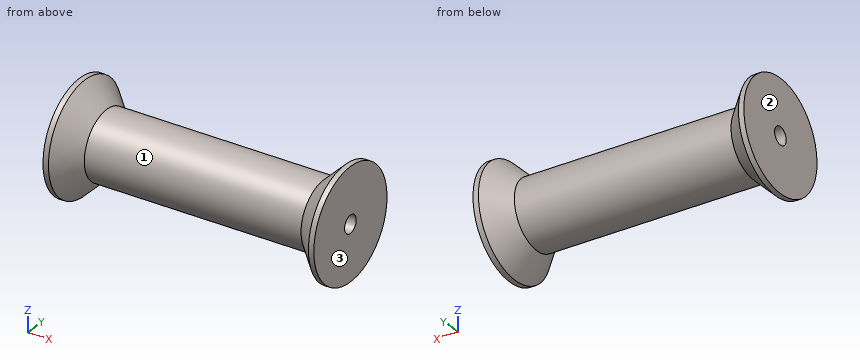
```python
from build123d import *


with BuildPart() as part:
    # Sketch1 → Revolve1 (revolve)
    with BuildSketch(Plane.XY, mode=Mode.PRIVATE) as revolve1_sk:
        with BuildLine():
            Line((0, 3.25), (10, 3.25))
            ThreePointArc((10, 3.25), (20.351145141, 7.537584704), (31.459292144, 9))
            Line((31.459292144, 9), (68.540707856, 9))
            ThreePointArc((68.540707856, 9), (79.648854859, 7.537584704), (90, 3.25))
            Line((90, 3.25), (100, 3.25))
            Line((100, 3.25), (100, 20.5))
            Line((100, 20.5), (98, 20.5))
            Line((98, 20.5), (90, 12.5))
            Line((90, 12.5), (10, 12.5))
            Line((10, 12.5), (2, 20.5))
            Line((2, 20.5), (0, 20.5))
            Line((0, 20.5), (0, 3.25))
        make_face()
    revolve(revolve1_sk.sketch.rotate(Axis((0, 0, 0), (1, 0, 0)), 90), axis=Axis((0, 0, 0), (1, 0, 0)))


solid = part.part
```
Model file for the job. Use its own axes, mm. Face numbers are marked on the shaded views. Round coordinates to 2 decimals unless told otherwise and drop trailing zeros. Write each loop counter-clockwise with the first axis right and the second up, starting at its lowest first coordinate (ties: lowest second). Pieces come first, ordered by that corner, then holes. Notation, with made-up numbers: (8, 19.25) -> (50, 19.25) arc R11 cw to (50, 37.25) -> close; hole circle Ø7 at (85.25, -18). An arc over 180 degrees is marked (long way). Answer as CSV lines item,"result".
1. Pin check, flat tips, straight feed: pin 1 Ø10 at (x, y) = (34.5, -15) entering from -Z; pin 2 Ø1.5 at (x, y) = (87.5, -8) entering from +Z; pin 3 Ø4 at (x, z) = (15, -2.5) entering from +Y. Stop position of each tip, or through.
Resolved:
pin 1,"z = -7.5"
pin 2,"z = 10.18"
pin 3,"y = 12.49"
2. Drill centre lines: line 1 (Y direction, x = 40, z = 0); line 2 (X direction, y = 16, z = 6.5); line 3 (Z direction, x = 19.5, y = 6.5). Where is each one in solid material? Low to high.
Resolved:
line 1,"-12.5 to -9, 9 to 12.5"
line 2,"0 to 5.23, 94.77 to 100"
line 3,"-10.68 to -3.32, 3.32 to 10.68"
3. Mould opens along X. For the marked faces 1, 2 and 3 say: +X half, -X half, draft (parallel to the pull), parting line (faces both ways), or undercut.
Resolved:
face 1,"undercut"
face 2,"-X half"
face 3,"+X half"
4. Slice it at A-A, the plane x = 67. List the corners of the cut face in (y, z).
Resolved:
outline,"circle Ø25 at (0, 0); hole circle Ø18 at (0, 0)"
